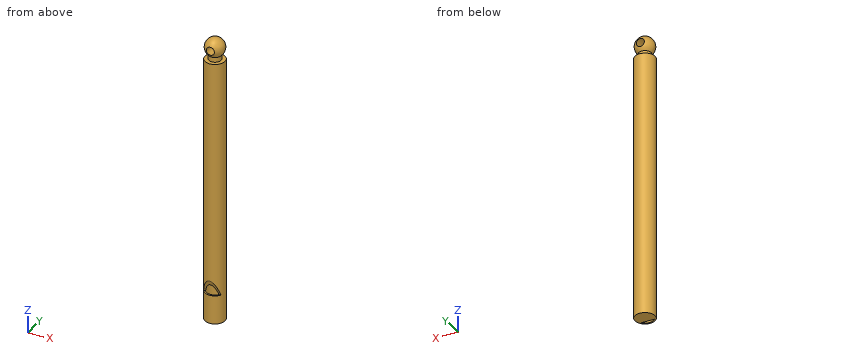
```python
from build123d import *

# Parameters (mm, degrees)
F2_R     = 1.25
F3_DEPTH = 12.7
F5_DEPTH = 12.7
F6_R     = 2.6
F7_DEPTH = 81
F9_DEPTH = 0.5


with BuildPart() as f1:
    # F0 (on Front) → F1 (revolve)
    with BuildSketch(Plane.XZ):
        with BuildLine():
            Line((0, -86.066867), (0, 2.965))
            ThreePointArc((0, 2.965), (-2.792977, 0.995242), (-1.875, -2.296867))
            Line((-1.875, -2.296867), (-1.875, -3.796867))
            Line((-1.875, -3.796867), (-3.1, -3.796867))
            Line((-3.1, -3.796867), (-3.1, -86.066867))
            Line((-3.1, -86.066867), (0, -86.066867))
        make_face()
    revolve(axis=Axis((0, 0, -41.550934), (0, 0, 1)))

    # F2 (on Front) → F3 (cut, symmetric)
    with BuildSketch(Plane.XZ):
        Circle(F2_R)
    extrude(amount=F3_DEPTH, both=True, mode=Mode.SUBTRACT)

    # F4 (on Right) → F5 (cut, symmetric)
    with BuildSketch(Plane.YZ):
        Polygon((-3.100019, -72.666867), (-3.100019, -77.166867), (-1.560019, -77.166867), align=None)
    extrude(amount=F5_DEPTH, both=True, mode=Mode.SUBTRACT)

    # F6 (on face) → F7 (cut)
    with BuildSketch(Plane(origin=(0, 0, -86.066867), x_dir=(1, 0, 0), z_dir=(0, 0, -1))):
        Circle(F6_R)
    extrude(amount=-F7_DEPTH, mode=Mode.SUBTRACT)

    # F8 (on face) → F9 (join)
    with BuildSketch(Plane(origin=(0, 0, -86.066867), x_dir=(1, 0, 0), z_dir=(0, 0, -1))):
        with BuildLine():
            ThreePointArc((-2, 1.661325), (-0.883176, -2.445404), (2.6, 0))
            ThreePointArc((2.6, 0), (2.445404, 0.883176), (2, 1.661325))
            Line((2, 1.661325), (-2, 1.661325))
        make_face()
    extrude(amount=-F9_DEPTH)


solid = f1.part
```
For this review, take the finished solid that the model builds, in its own axes (mm). Round coordinates to 2 decimals unless told otherwise and drop trailing zeros. Loops run counter-clockwise (first coordinate to the right, second up) from the corner with the lowest first, then second, coordinate; pieces in that order, holes last.
(1) Wall thickness on line 1 along Z through (x, y) = (0, 1.3); line 2 along X through (y, z) = (0, -41); line 3 along Z through (x, y) = (1, 1.5): over which ranges is each line inside the solid? List them lowest first.
Returned:
line 1: z = -86.07 to -85.57, -5.07 to -1.25, 1.25 to 2.66
line 2: x = -3.1 to -2.6, 2.6 to 3.1
line 3: z = -86.07 to -85.57, -5.07 to -0.75, 0.75 to 2.35
(2) We need section A-A (z = -70.5). Give the boundary of the cut face in (x, y).
Returned:
outline: circle Ø6.2 at (0, 0); hole circle Ø5.2 at (0, 0)
(3) Clearance check with flat-ended pins moving along their axes: P1, Ø0.5, axis at x = -0.5, y = -2.5, coming from the +Z side; P2, Ø2, axis at x = -0.5, y = 2, coming from the +Z side; P3, Ø3, axis at x = 1, y = 0.5, coming from the +Z side (3 decimals); P4, Ø1, axis at x = -1, z = -11, coming from the -Y side. State where each tip first meets the part, or that it passes through.
Returned:
P1: stops at z = 1.87
P2: stops at z = 2.77
P3: stops at z = 2.965
P4: stops at y = -3.06
